Autodesk Inventor part; units mm, degrees
ref_plane "YZ Plane" through (0, 0, 0) normal (1, 0, 0) x (0, 1, 0)
ref_plane "XZ Plane" through (0, 0, 0) normal (0, 1, 0) x (-1, 0, 0)
ref_plane "XY Plane" through (0, 0, 0) normal (0, 0, 1) x (1, 0, 0)
sketch "Skizze1" plane through (0, 0, 0) normal (0, 0, 1) x (1, 0, 0)
  circle A0 centre (0, 0) radius 4.2
  circle A1 centre (0, 0) radius 12
  dimension "d0" = 24
  dimension "d1" = 8.4
extrude "Extrusion1" add sketch "Skizze1" along normal mid plane 2
chamfer "Fase1" distance 0.2 angle 45 4 edges at (-12, 0, 1) (-12, 0, -1) (-4.2, 0, 1) (-4.2, 0, -1)
properties part number "900-80-WASHERS-DIN9021-M8" material "Edelstahl"
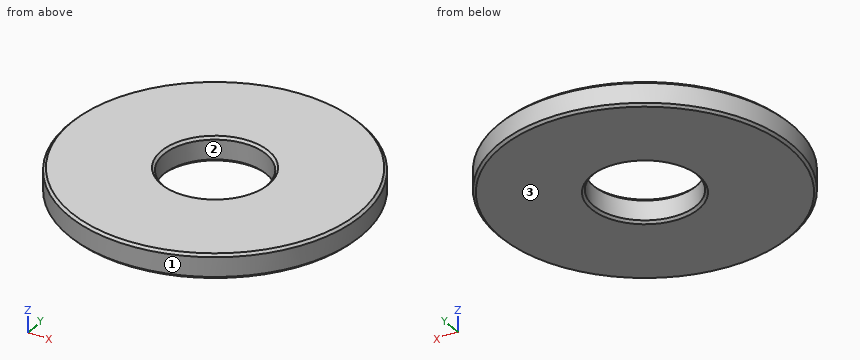
Read the model definition and answer for the solid it produces. Units are mm, in the model's axes. Face numbers are marked on the shaded views. Give positions to 0.01 mm unless a question says otherwise; leave off trailing zeros. Order: outer loops, then holes, each group sorted by start corner. A loop starts at its lowest first (then second) coordinate and runs counter-clockwise, first axis right, second up. Notation, with made-up numbers: (12.25, 4.25) -> (44.25, 4.25) arc R8 cw to (44.25, 14.25) -> close; hole circle Ø2 at (66.5, 30.25). An arc over 180 degrees is marked (long way). One line per item, written item: value. Start each with the question number.
(1) The part is cut by section A-A (y = 0). Determine the outline of the cut face in (x, z).
(2) For a pull along Y with two mould halves and no side action, classify the marked faces 1, 2 and 3 as released by +Y, released by -Y, zero draft, split by the parting line, or undercut.
(3) Straight lines are drawn through the part: L1, parallel to Y at x = 0, z = -0.25; L2, parallel to Y at x = 2, z = 0.2; L3, parallel to X at y = -2.25, z = 0.05. For each, find the intervals that lie inside material, in ascending order.
(4) The part is cut by section C-C (z = 0.2). Determine the outline of the cut face in (x, y), and give its area (3 significant figures).
Taken from the geometry:
1. outline: (-12, -0.8) -> (-11.8, -1) -> (-4.4, -1) -> (-4.2, -0.8) -> (-4.2, 0.8) -> (-4.4, 1) -> (-11.8, 1) -> (-12, 0.8) -> close; (4.2, -0.8) -> (4.4, -1) -> (11.8, -1) -> (12, -0.8) -> (12, 0.8) -> (11.8, 1) -> (4.4, 1) -> (4.2, 0.8) -> close
2. face 1: split by the parting line
2. face 2: undercut
2. face 3: zero draft
3. L1: -12 to -4.2, 4.2 to 12
3. L2: -11.83 to -3.69, 3.69 to 11.83
3. L3: -11.79 to -3.55, 3.55 to 11.79
4. outline: circle Ø24 at (0, 0); hole circle Ø8.4 at (0, 0)
4. area: 397 mm^2
